The model under review builds one solid part; all positions refer to its coordinate system, in mm. Face numbers are marked on the shaded views. A direction names the side the tool comes from. Coordinates: 2 decimals unless noted, no trailing zeros. Order: outer loops, then holes, each group sorted by start corner. A loop starts at its lowest first (then second) coordinate and runs counter-clockwise, first axis right, second up. Notation, with made-up numbers: M 38.5,58 L 96.5,58 A21 ccw 96.5,65 Z; hole C 55.25,27.5 d4. An arc over 180 degrees is marked long. Answer in a Markdown table with one row per item.
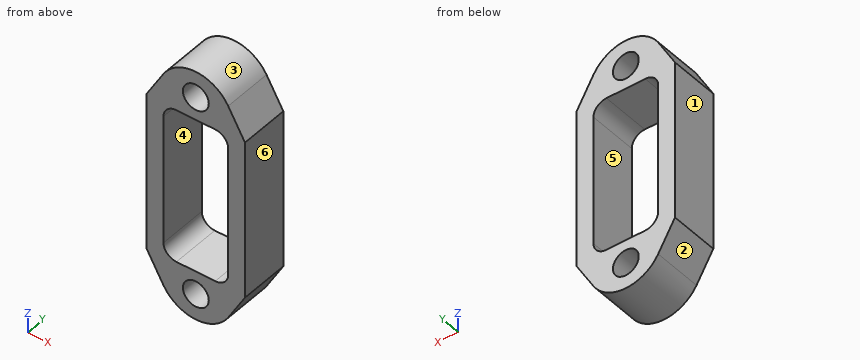
from build123d import *

# Parameters (mm, degrees)
F0_R     = 5
F1_DEPTH = 19


with BuildPart() as f1:
    # F0 (on Front) → F1 (new body)
    with BuildSketch(Plane.XZ):
        with BuildLine():
            Line((-12.5, 41.820371), (-19, 30.677514))
            Line((-19, 30.677514), (-19, 0))
            Line((-19, 0), (-19, -30.677514))
            Line((-19, -30.677514), (-12.5, -41.820371))
            ThreePointArc((-12.5, -41.820371), (0, -49), (12.5, -41.820371))
            Line((12.5, -41.820371), (19, -30.677514))
            Line((19, -30.677514), (19, 0))
            Line((19, 0), (19, 30.677514))
            Line((19, 30.677514), (12.5, 41.820371))
            ThreePointArc((12.5, 41.820371), (0, 49), (-12.5, 41.820371))
        make_face()
        with Locations((0, -38.9)):
            Circle(F0_R, mode=Mode.SUBTRACT)
        with BuildLine():
            Line((-12.5, -25), (-12.5, 0))
            Line((-12.5, 0), (-12.5, 25))
            ThreePointArc((-12.5, 25), (-11.035534, 28.535534), (-7.5, 30))
            Line((-7.5, 30), (0, 30))
            Line((0, 30), (7.5, 30))
            ThreePointArc((7.5, 30), (11.035534, 28.535534), (12.5, 25))
            Line((12.5, 25), (12.5, 0))
            Line((12.5, 0), (12.5, -25))
            ThreePointArc((12.5, -25), (11.035534, -28.535534), (7.5, -30))
            Line((7.5, -30), (0, -30))
            Line((0, -30), (-7.5, -30))
            ThreePointArc((-7.5, -30), (-11.035534, -28.535534), (-12.5, -25))
        make_face(mode=Mode.SUBTRACT)
        with Locations((0, 38.9)):
            Circle(F0_R, mode=Mode.SUBTRACT)
    extrude(amount=F1_DEPTH)


solid = f1.part
(1) Take a section at A-A (x = 0). Write out the cut boundary in (y, z).
Report:
| item | result |
|---|---|
| outline | M -19,-49 L 0,-49 L 0,-43.9 L -19,-43.9 Z; M -19,-33.9 L 0,-33.9 L 0,-30 L -19,-30 Z; M -19,30 L 0,30 L 0,33.9 L -19,33.9 Z; M -19,43.9 L 0,43.9 L 0,49 L -19,49 Z |
(2) Insertion check: P1, Ø13, axis at x = 0, z = 38.9, coming from the +Y side; P2, Ø1, axis at x = -5, y = -8, coming from the +Z side; P3, Ø4.5, axis at x = -2.5, y = -6.5, coming from the -Z side; P4, Ø10, axis at x = -12, y = -10.5, coming from the -Z side. Each pin has a flat end and moves straight along its axis. Give the tip position at first contact, or say it passes through.
Report:
| item | result |
|---|---|
| P1 | y = 0 |
| P2 | z = 48.28 |
| P3 | z = -49 |
| P4 | z = -47.19 |
(3) Take a section at B-B (z = 16). Write out the cut boundary in (x, y), then the cut area to 3 significant figures.
Report:
| item | result |
|---|---|
| outline | M -19,-19 L -12.5,-19 L -12.5,0 L -19,0 Z; M 12.5,-19 L 19,-19 L 19,0 L 12.5,0 Z |
| area | 247 mm^2 |
(4) Machinability: for the marked faces 5 and 6, which of the approach directions +Z, -Z, +X, -X, +Y, -Y give a long, thin tool a straight path to every point of the face, cutting with its end or side? Answer none if there is none.
Report:
| item | result |
|---|---|
| face 5 | +Y, -Y |
| face 6 | +Z, -Z, +X, +Y, -Y |
(5) To check wall thickness, follow line 1 (Z direction, x = 1.5, y = -18); line 2 (X direction, y = -6.75, z = -8); line 3 (Z direction, x = -3, y = -12.25). State the ranges of each line that lie inside material, in increasing order. Write a range as [from, to].
Report:
| item | result |
|---|---|
| line 1 | [-48.92, -43.67], [-34.13, -30], [30, 34.13], [43.67, 48.92] |
| line 2 | [-19, -12.5], [12.5, 19] |
| line 3 | [-48.69, -42.9], [-34.9, -30], [30, 34.9], [42.9, 48.69] |
(6) Take a section at C-C (y = -2.25). Write out the cut boundary in (x, z).
Report:
| item | result |
|---|---|
| outline | M -19,-30.68 L -12.5,-41.82 A14.47 ccw 12.5,-41.82 L 19,-30.68 L 19,30.68 L 12.5,41.82 A14.47 ccw -12.5,41.82 L -19,30.68 Z; hole M -12.5,-25 A5 ccw -7.5,-30 L 7.5,-30 A5 ccw 12.5,-25 L 12.5,25 A5 ccw 7.5,30 L -7.5,30 A5 ccw -12.5,25 Z; hole C 0,-38.9 d10; hole C 0,38.9 d10 |
(7) The part is to be moulded in two halves that separate along Z. For the marked faces 1, 2, 3 and 4, say which applies: +Z half, -Z half, draft (parallel to the pull), parting line (faces both ways), or undercut.
Report:
| item | result |
|---|---|
| face 1 | draft |
| face 2 | -Z half |
| face 3 | +Z half |
| face 4 | undercut |
(8) Take a section at D-D (x = 9). Write out the cut boundary in (y, z), then the cut area to 3 significant figures.
Report:
| item | result |
|---|---|
| outline | M -19,-45.86 L 0,-45.86 L 0,-29.77 L -19,-29.77 Z; M -19,29.77 L 0,29.77 L 0,45.86 L -19,45.86 Z |
| area | 611 mm^2 |
